Could you check a few things on this drawing? It's one solid part, dimensions in mm from its lowest x, y, z. Coordinates: 2 decimals unless noted, no trailing zeros. Write each loop counter-clockwise with the first axis right and the second up, starting at its lowest first coordinate (ties: lowest second). Pieces come first, ordered by that corner, then holes. Notation, with made-up numbers: M 89,9.25 L 146,9.25 A18 ccw 146,39.25 Z; hole C -8,74.5 d11. An arc over 180 degrees is marked long. Use a Markdown table: item, result.
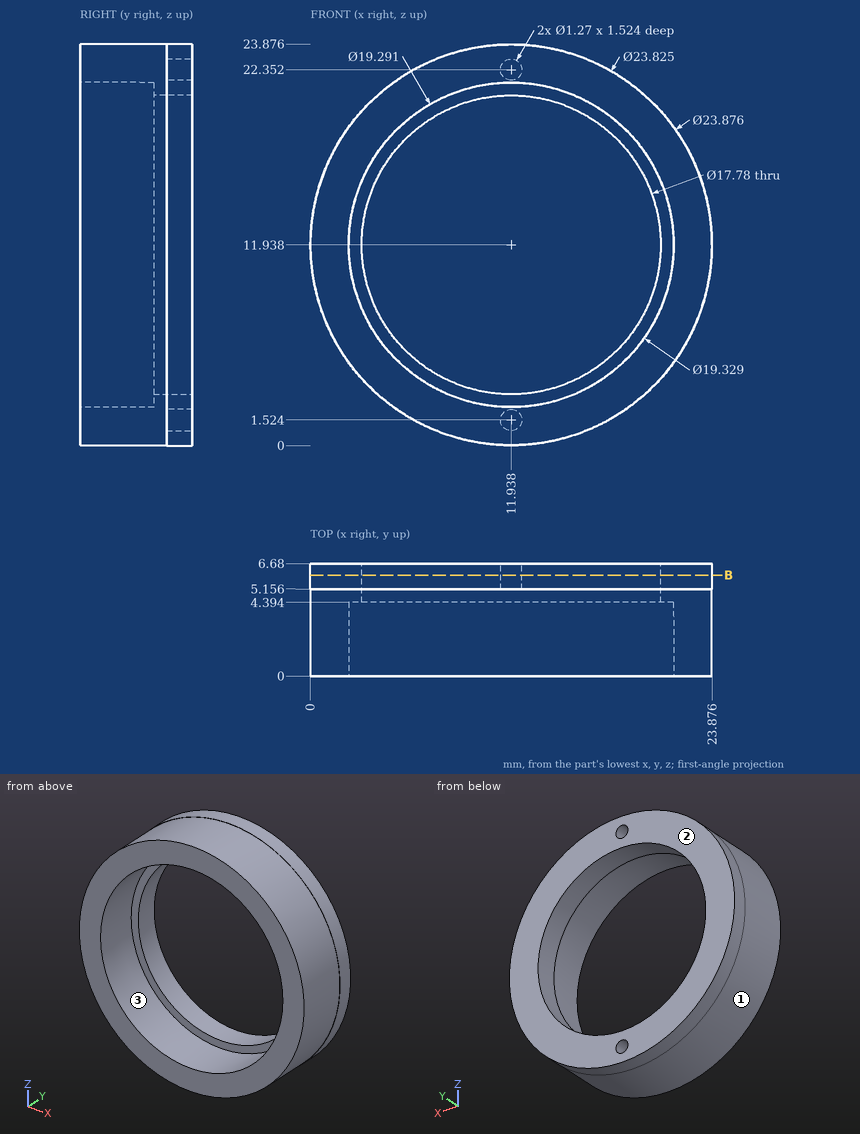
1. We'd pull the mould along Z, two halves only. Please class the marked faces 1, 2 and 3: +Z half, -Z half, draft (parallel to the pull), parting line (faces both ways), or undercut.
Answers follow:
| item | result |
|---|---|
| face 1 | parting line |
| face 2 | draft |
| face 3 | undercut |
2. Will these pins go through, and if not, where does the flat tip stop? pin 1 Ø6 at (x, z) = (8, 8) entering from -Y; pin 2 Ø1 at (x, y) = (17, 1) entering from -Z; pin 3 Ø4 at (x, y) = (19, 3) entering from +Z; pin 4 Ø1.5 at (y, z) = (3.5, 15) entering from +X.
Answers follow:
| item | result |
|---|---|
| pin 1 | passes through |
| pin 2 | stops at z = 0.93 |
| pin 3 | stops at z = 22.72 |
| pin 4 | stops at x = 23.62 |
3. Suppose I cut it at B-B on y = 6. Write out the boundary of the cut face in (x, z) (1 decimal).
Answers follow:
| item | result |
|---|---|
| outline | C 11.9,11.9 d23.9; hole C 11.9,11.9 d17.8; hole C 11.9,1.5 d1.3; hole C 11.9,22.4 d1.3 |
4. I need wall thicknesses on probe 1 along Z at (x, y) = (9.25, 5) (1 decimal); probe 2 along X at (y, z) = (1.75, 8.5) (1 decimal); probe 3 along X at (y, z) = (0.75, 15.75) (1 decimal). Which ranges of each line are inside material? Lowest first, please.
Answers follow:
| item | result |
|---|---|
| probe 1 | z = 0.3 to 3.5, 20.4 to 23.5 |
| probe 2 | x = 0.5 to 2.9, 21 to 23.3 |
| probe 3 | x = 0.7 to 3.1, 20.8 to 23.2 |
